Geometry check sheet. Reference: the model listing, model coordinates, mm. Face numbers are marked on the shaded views. A direction names the side the tool comes from. Coordinates: 2 decimals unless noted, no trailing zeros. Order: outer loops, then holes, each group sorted by start corner. A loop starts at its lowest first (then second) coordinate and runs counter-clockwise, first axis right, second up. Notation, with made-up numbers: M 86,69.25 L 118,69.25 A22 ccw 118,86.25 Z; hole C 71.5,22 d3. An arc over 180 degrees is marked long. One line per item, written item: value. Start each with the question number.
1) Sectioned sample at B-B, the plane x = 4.5. Enter the section's corners in (y, z), then the cut area to 3 significant figures.
2) Sectioned sample at A-A, the plane x = 23. Enter the section's corners in (y, z).
3) Draft check along Y on the marked faces 4, 5, 6 and 7. Enter one of: pulls with the +Y half, pulls with the -Y half, needs draft (parallel to the pull), parting line crosses it, or undercut.
4) Thickness scan on L1, parallel to X at y = 12, z = 43; L2, parallel to X at y = 4.5, z = 46; L3, parallel to Z at x = -17, y = -1. Record the ranges inside material, lowest first. Write a range as from..to.
5) Go/stop test with flat-tipped pins: P1, Ø4, axis at x = -17, z = 36.5, coming from the -Y side; P2, Ø3, axis at x = 24.5, z = 25.5, coming from the -Y side; P3, Ø10, axis at x = 19, y = -16.5, coming from the -Z side; P4, Ø12, axis at x = 19, z = 31.5, coming from the -Y side. Record where each tip stops, or that it passes through.
6) Access from +Z, -Z, +X, -X, +Y, -Y to the whole of each face (thin tool, end or side, straight path). Record for the marked faces 1, 2 and 3.
```python
from build123d import *

# Parameters (mm, degrees)
F0_W     = 62.4118931592
F0_H     = 47.6785954088
F1_DEPTH = 59.436
F3_DEPTH = 62.4128931592
F4_R     = 11.5061278917
F5_DEPTH = 9.525
F6_R     = 6.35


with BuildPart() as f1:
    # F0 (on Top) → F1 (new body)
    with BuildSketch(Plane.XY):
        Rectangle(F0_W, F0_H)
    extrude(amount=F1_DEPTH)

    # F2 (on face) → F3 (cut, through all)
    with BuildSketch(Plane(origin=(-31.2059465796, 0, 0), x_dir=(0, -1, 0), z_dir=(-1, 0, 0))):
        Polygon((23.8392977044, 59.436), (-5.6998856858, 59.436), (0, 27.1103419363), (23.8392977044, 31.3138533228), align=None)
    extrude(amount=-F3_DEPTH, mode=Mode.SUBTRACT)

    # F4 (on face) → F5 (cut)
    with BuildSketch(Plane(origin=(0, -4.6361415173, 0.8174768359), x_dir=(1, 0, 0), z_dir=(0, -0.984807753, 0.1736481777))):
        with Locations((0, 42.3641316593)):
            Circle(F4_R)
    extrude(amount=-F5_DEPTH, mode=Mode.SUBTRACT)

    # F6
    f6_edges = [f1.edges().sort_by_distance(p)[0] for p in [
        (0, 23.839298, 59.436),
        (31.205947, 14.769592, 59.436),
        (0, 5.699886, 59.436),
        (-31.205947, 14.769592, 59.436),
        (-31.205947, -23.839298, 15.656927),
        (31.205947, -23.839298, 15.656927),
        (0, -23.839298, 31.313853),
        (-31.205947, -11.919649, 29.212098),
        (-31.205947, 2.849943, 43.273171),
        (31.205947, -11.919649, 29.212098),
        (31.205947, 2.849943, 43.273171),
        (31.205947, 23.839298, 29.718),
        (-31.205947, 23.839298, 29.718),
    ]]
    fillet(f6_edges, radius=F6_R)


solid = f1.part
```
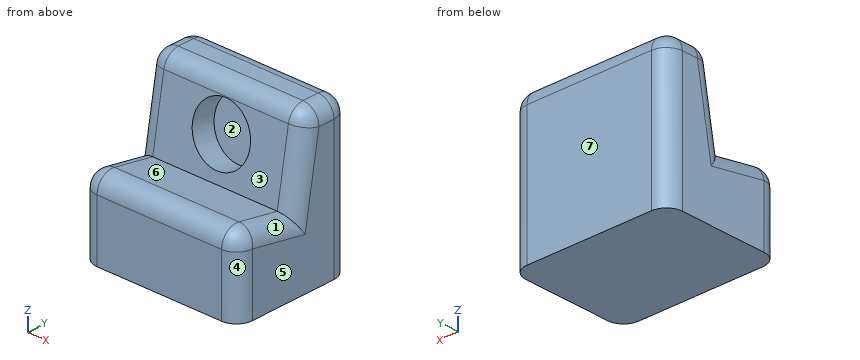
Final values:
1. outline: M -23.84,0 L 23.84,0 L 23.84,53.09 A6.35 ccw 17.49,59.44 L 11.03,59.44 A6.35 ccw 4.77,54.19 L 4.56,52.97 L 13.94,51.31 L 10.26,30.46 L 0.88,32.11 L 0,27.11 L -16.39,30 A6.35 ccw -23.84,23.75 Z
1. area: 1,790 mm^2
2. outline: M -23.84,0 L 23.84,0 L 23.84,53.09 A6.35 ccw 17.49,59.44 L 11.03,59.44 A6.35 ccw 4.77,54.19 L 0,27.11 L -16.39,30 A6.35 ccw -23.84,23.75 Z
3. face 4: pulls with the -Y half
3. face 5: needs draft
3. face 6: undercut
3. face 7: pulls with the +Y half
4. L1: x = -31.21..-11.32, 11.32..31.21
4. L2: x = -28.5..-10.89, 10.89..28.5
4. L3: z = 0..27.29
5. P1: stops at y = 1.3
5. P2: stops at y = -23.83
5. P3: stops at z = 0
5. P4: stops at y = -23.59
6. face 1: +Z, +X
6. face 2: none
6. face 3: +Z, +X, -X
